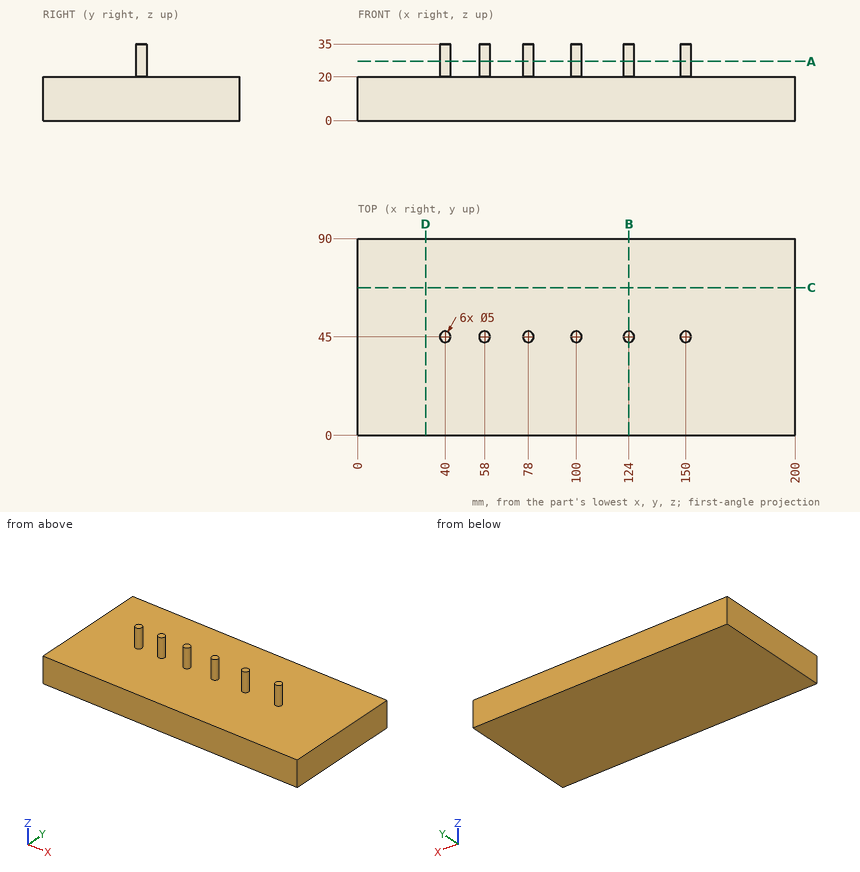
Source: three-view drawing plus pictorial views. Frame: mm from the lowest corner of the part. Round coordinates to 2 decimals unless told otherwise and drop trailing zeros. Loops run counter-clockwise (first coordinate to the right, second up) from the corner with the lowest first, then second, coordinate; pieces in that order, holes last.
Q1. Material intervals for L1, parallel to Z at x = 91.5, y = 79, sorted ascending.
Q2. Section B-B on x = 124. Return loops of the section in (y, z), plus the area to 4 significant figures.
Q3. Section A-A on z = 27. Return loops of the section in (x, y), plus the area to 3 significant figures.
Q4. Pin query (flat end, axial travel): P1, Ø8, axis at y = 73, z = 27.5, coming from the -X side; P2, Ø2, axis at x = 164, y = 57, coming from the +Z side. Return the tip coordinate at first contact, or that it passes through.
Q5. Section D-D on x = 31. Return loops of the section in (y, z), plus the area to 3 significant figures.
Q6. Section C-C on y = 67.5. Return loops of the section in (x, z), plus the area to 3 significant figures.
Evaluation:
1. L1: z = 0 to 20
2. outline: (0, 0) - (90, 0) - (90, 20) - (47.5, 20) - (47.5, 35) - (42.5, 35) - (42.5, 20) - (0, 20) - close
2. area: 1,875 mm2
3. outline: circle Ø5 at (40, 45); circle Ø5 at (58, 45); circle Ø5 at (78, 45); circle Ø5 at (100, 45); circle Ø5 at (124, 45); circle Ø5 at (150, 45)
3. area: 118 mm2
4. P1: passes through
4. P2: stops at z = 20
5. outline: (0, 0) - (90, 0) - (90, 20) - (0, 20) - close
5. area: 1,800 mm2
6. outline: (0, 0) - (200, 0) - (200, 20) - (0, 20) - close
6. area: 4,000 mm2
